```python
from build123d import *

# Parameters (mm, degrees)
SKETCH2_R           = 2.5
BOSS_EXTRUDE1_DEPTH = 32
BOSS_EXTRUDE2_DEPTH = 4
BOSS_EXTRUDE2_TAPER = 20
CUT_EXTRUDE1_DEPTH  = 6
CUT_EXTRUDE2_DEPTH  = 6
SKETCH6_R           = 5
BOSS_EXTRUDE3_DEPTH = 4
FILLET1_R           = 4


with BuildPart() as part:
    # Sketch2 → Boss-Extrude1 (new body)
    with BuildSketch(Plane.XY):
        Circle(SKETCH2_R)
    extrude(amount=BOSS_EXTRUDE1_DEPTH)

    # Sketch3 → Boss-Extrude2 (add)
    with BuildSketch(Plane(origin=(0, 0, 0), x_dir=(-1, 0, 0), z_dir=(0, 0, -1))):
        with BuildLine():
            ThreePointArc((2.910177967, 1.944444444), (0, 3.5), (-2.910177967, 1.944444444))
            ThreePointArc((-2.910177967, 1.944444444), (-3.5, 0), (-2.910177967, -1.944444444))
            ThreePointArc((-2.910177967, -1.944444444), (0, -3.5), (2.910177967, -1.944444444))
            ThreePointArc((2.910177967, -1.944444444), (3.349300142, -1.015966809), (3.5, 0))
            ThreePointArc((3.5, 0), (3.349300142, 1.015966809), (2.910177967, 1.944444444))
        make_face()
    extrude(amount=BOSS_EXTRUDE2_DEPTH, taper=BOSS_EXTRUDE2_TAPER)

    # Sketch4 → Cut-Extrude1 (cut)
    with BuildSketch(Plane.XY):
        Polygon((4.702019348, 2.5), (-6.119643092, 2.5), (-4.730091105, -2.5), (5.600315582, -2.5), (7.628500047, -1.168486898), (5.144149526, -5.126604677), (-5.530136189, -4.719564196), (-7.70569738, 3.519496572), (-2.540721352, 4.883331809), (4.16163802, 4.824833286), (4.784967696, 2.464223482), align=None)
    extrude(amount=-CUT_EXTRUDE1_DEPTH, mode=Mode.SUBTRACT)

    # Sketch5 → Cut-Extrude2 (cut)
    with BuildSketch(Plane(origin=(0, 2.5, 0), x_dir=(1, 0, 0), z_dir=(0, 1, 0))):
        with BuildLine():
            Line((1.25, 19), (1.25, -11))
            ThreePointArc((1.25, -11), (0, -12.25), (-1.25, -11))
            Line((-1.25, -11), (-1.25, 19))
            ThreePointArc((-1.25, 19), (0, 20.25), (1.25, 19))
        make_face()
    extrude(amount=-CUT_EXTRUDE2_DEPTH, mode=Mode.SUBTRACT)

    # Sketch6 → Boss-Extrude3 (add)
    with BuildSketch(Plane.XY.offset(32)):
        Circle(SKETCH6_R)
    extrude(amount=BOSS_EXTRUDE3_DEPTH)

    # Fillet1
    fillet1_edges = [part.edges().sort_by_distance(p)[0] for p in [
        (-5, 0, 36),
    ]]
    fillet(fillet1_edges, radius=FILLET1_R - 0.0001)  # a hair under: the kernel refuses the full size


solid = part.part
```
For this review, take the finished solid that the model builds, in its own axes (mm). A direction names the side the tool comes from. Coordinates: 2 decimals unless noted, no trailing zeros. Write each loop counter-clockwise with the first axis right and the second up, starting at its lowest first coordinate (ties: lowest second). Pieces come first, ordered by that corner, then holes. Notation, with made-up numbers: (39, 52) - (48, 52) arc R10 ccw to (48, 69) - close; hole circle Ø5 at (14.5, -4.75). An arc over 180 degrees is marked (long way). Answer in a Markdown table with one row per item. Add a question column.
Q1. We need section B-B, the plane z = 11.5. State the section outline as (x, y) points, and give its area (3 significant figures).
Q2. Draft analysis for pull direction Z (two halves, no side actions). For faces 6 (the flat face through (-1.7, 2.5, -0.7)), 7 (the flat face through (0, 0, 36)), 8 (the flat face through (2, -2, 32)), state which applies: +Z half, -Z half, draft (parallel to the pull), parting line (faces both ways), or undercut.
Q3. Tool access review of faces 1 (the flat face through (-3, 0, 0)), 2 (the flat face through (1.7, 2.5, -0.7)), 3 (the flat face through (3, 0, 0)), 4 (the flat face through (-1.25, 0, 4)), 5 (the flat face through (-1.7, -2.5, -0.7)): name each direction out of +Z, -Z, +X, -X, +Y, -Y from which nothing blocks a thin tool from reaching the whole face with its end or side.
Q4. For probe 1 along X at (y, z) = (1, 7); probe 2 along X at (y, z) = (-0.25, 7); probe 3 along Z at (x, y) = (0.25, -1.25), list the stretches that pass through material, from the lowest coordinate up.
Q5. We need section A-A, the plane z = 18. State the section outline as (x, y) points.
Q6. For P1, Ø1.5, axis at x = 0, z = 6, coming from the -Y side; P2, Ø5.5, axis at y = 1, z = 4.5, coming from the +X side; P3, Ø1, axis at x = -1.5, z = -1.5, coming from the -Y side; P4, Ø1.3, axis at x = 1.5, z = -1, coming from the +Y side, all flat-tipped, find the tip position at first contact; note any pin that passes through.
Answer list:
| question | item | result |
|---|---|---|
| 1 | outline | (-1.15, -2.22) - (-1.15, 2.22) arc R2.5 ccw to start; (1.15, -2.22) arc R2.5 ccw to (1.15, 2.22) - close |
| 1 | area | 8.59 mm2 |
| 2 | face 6 | draft |
| 2 | face 7 | +Z half |
| 2 | face 8 | undercut |
| 3 | face 1 | -X |
| 3 | face 2 | -Z, +X, -X, +Y |
| 3 | face 3 | +X |
| 3 | face 4 | -Z, +Y, -Y |
| 3 | face 5 | -Z, +X, -X, -Y |
| 4 | probe 1 | x = -2.29 to -1.25, 1.25 to 2.29 |
| 4 | probe 2 | x = -2.49 to -1.25, 1.25 to 2.49 |
| 4 | probe 3 | z = 12.22 to 35.99 |
| 5 | outline | circle Ø5 at (0, 0) |
| 6 | P1 | passes through |
| 6 | P2 | stops at x = 2.5 |
| 6 | P3 | stops at y = -2.5 |
| 6 | P4 | stops at y = 2.5 |
